```python
from build123d import *

# Parameters (mm, degrees)
SKETCH1_W           = 100
SKETCH1_H           = 200
BOSS_EXTRUDE1_DEPTH = 10
SKETCH2_W           = 50
SKETCH2_H           = 40
BOSS_EXTRUDE2_DEPTH = 25
SKETCH4_R           = 12.5
CUT_EXTRUDE1_DEPTH  = 25


with BuildPart() as part:
    # Sketch1 → Boss-Extrude1 (new body)
    with BuildSketch(Plane(origin=(0, 0, 0), x_dir=(1, 0, 0), z_dir=(0, 1, 0))):
        with Locations((50, 100)):
            Rectangle(SKETCH1_W, SKETCH1_H)
    extrude(amount=BOSS_EXTRUDE1_DEPTH)

    # Sketch2 → Boss-Extrude2 (add)
    with BuildSketch(Plane(origin=(0, 10, 0), x_dir=(1, 0, 0), z_dir=(0, 1, 0))):
        with Locations((25, 20)):
            Rectangle(SKETCH2_W, SKETCH2_H)
    extrude(amount=BOSS_EXTRUDE2_DEPTH)

    # Sketch4 → Cut-Extrude1 (cut)
    with BuildSketch(Plane(origin=(0, 10, 0), x_dir=(1, 0, 0), z_dir=(0, 1, 0))):
        with Locations((35, 170)):
            Circle(SKETCH4_R)
    extrude(amount=-CUT_EXTRUDE1_DEPTH, mode=Mode.SUBTRACT)


solid = part.part
```
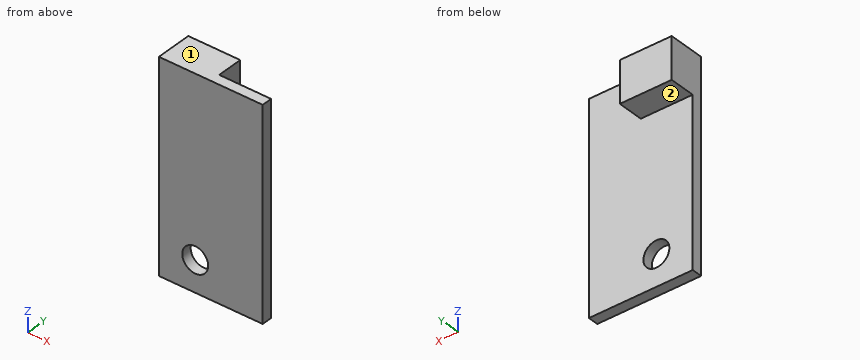
CAD build for the part. Positions are in the model's coordinates, mm. Face numbers are marked on the shaded views. A direction names the side the tool comes from. Round coordinates to 2 decimals unless told otherwise and drop trailing zeros. Order: outer loops, then holes, each group sorted by start corner. A loop starts at its lowest first (then second) coordinate and runs counter-clockwise, first axis right, second up.
Q1. Slice it at B-B (z = -170). Write the cut outline in (x, y), and give its area (3 significant figures).
Q2. Slice it at D-D (z = -21). Write the cut outline in (x, y).
Q3. Which spindle directions (+Z, -Z, +X, -X, +Y, -Y) get a long thin tool onto all of the face, cutting with end or side? Do the marked faces 1 and 2. Say none if no direction does.
Q4. Drop flat-ended pins along their axis: pin 1 (5 mm diameter, centred on x = 42, y = 31.5, fed in from -Z); pin 2 (2 mm diameter, centred on x = 67, z = -92, fed in from +Y); pin 3 (12.5 mm diameter, centred on y = 26.5, z = -12.5, fed in from +X). Give the stop position or say it passes through.
Q5. Slice it at C-C (y = 4.5). Write the cut outline in (x, z).
Q6. Wall check: L1, parallel to Z at x = 35, y = 7; L2, parallel to X at y = 5, z = -170; L3, parallel to X at y = 23, z = -15. Give the ranges that are in metal, low to high.
Q7. Slice it at A-A (x = 35). Write the cut outline in (y, z), and give its area (3 significant figures).
Results below:
1. outline: (0, 0) - (22.5, 0) - (22.5, 10) - (0, 10) - close; (47.5, 0) - (100, 0) - (100, 10) - (47.5, 10) - close
1. area: 750 mm2
2. outline: (0, 0) - (100, 0) - (100, 10) - (50, 10) - (50, 35) - (0, 35) - close
3. face 1: +Z, +X, -X, +Y, -Y
3. face 2: -Z, +X, -X, +Y
4. pin 1: stops at z = -40
4. pin 2: stops at y = 10
4. pin 3: stops at x = 50
5. outline: (0, -200) - (100, -200) - (100, 0) - (0, 0) - close; hole circle Ø25 at (35, -170)
6. L1: z = -200 to -182.5, -157.5 to 0
6. L2: x = 0 to 22.5, 47.5 to 100
6. L3: x = 0 to 50
7. outline: (0, -200) - (10, -200) - (10, -182.5) - (0, -182.5) - close; (0, -157.5) - (10, -157.5) - (10, -40) - (35, -40) - (35, 0) - (0, 0) - close
7. area: 2,750 mm2
